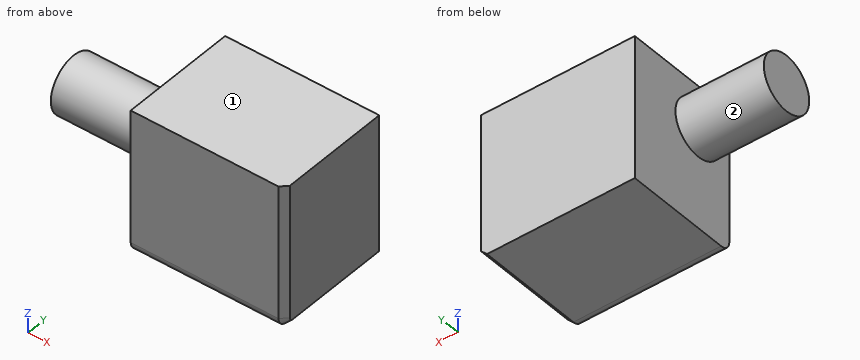
```python
from build123d import *

# Parameters (mm, degrees)
F0_W     = 125.304118
F0_H     = 116.59091
F1_DEPTH = 95.108278
F2_R     = 8.21097
F3_SIZE  = 5.08
F4_R     = 22.853538
F5_DEPTH = 71.891591


with BuildPart() as f1:
    # F0 (on Front) → F1 (new body)
    with BuildSketch(Plane.XZ):
        with Locations((1.244716, -1.867104)):
            Rectangle(F0_W, F0_H)
    extrude(amount=F1_DEPTH)

    # F2
    f2_edges = [f1.edges().sort_by_distance(p)[0] for p in [
        (1.244716, -95.108278, -60.162559),
    ]]
    fillet(f2_edges, radius=F2_R)

    # F3
    f3_edges = [f1.edges().sort_by_distance(p)[0] for p in [
        (63.896775, -95.108278, 2.238381),
    ]]
    chamfer(f3_edges, length=F3_SIZE)

    # F4 (on face) → F5 (join)
    with BuildSketch(Plane(origin=(-61.407343, 0, 0), x_dir=(0, -1, 0), z_dir=(-1, 0, 0))):
        with Locations((63.728884, 21.200262)):
            Circle(F4_R)
    extrude(amount=F5_DEPTH)


solid = f1.part
```
The listing builds one solid part. Answer for the finished solid, in the listing's coordinates (mm). Face numbers are marked on the shaded views. A direction names the side the tool comes from. Coordinates: 2 decimals unless noted, no trailing zeros. Write each loop counter-clockwise with the first axis right and the second up, starting at its lowest first coordinate (ties: lowest second). Pieces come first, ordered by that corner, then holes. Notation, with made-up numbers: M 46,14 L 62,14 A24 ccw 62,43 Z; hole C -37.75,42.25 d1. An arc over 180 degrees is marked long. Use a Markdown table: item, result. Add a question column.
1. Straight lines are drawn through the part: line 1 along X through (y, z) = (-38, 20.5); line 2 along Z through (x, y) = (-73.5, -64); line 3 along Y through (x, z) = (-117, 12). For each, find the intervals that lie inside material, in ascending order. Write a range as [from, to].
2. Section A-A (z = 34) is taken. Give the vertices of the cut face in (x, y).
3. Section C-C (x = -95) is taken. Give the vertices of the cut face in (y, z), plus the area to 3 significant figures.
4. Section D-D (z = 15) is taken. Give the vertices of the cut face in (x, y).
5. Which of the six approach directions +Z, -Z, +X, -X, +Y, -Y give full straight-line access (tool end or side, diameter ignored) to the marked faces 1 and 2?
6. Given P1, Ø3, axis at x = -88, z = 19.5, coming from the +Y side; P2, Ø12, axis at y = -63, z = -24, coming from the -X side, each flat-ended and moving along its own axis, determine where each tip first touches the part or whether it passes through.
7. Section B-B (y = -6.5) is taken. Give the vertices of the cut face in (x, z).
Data:
| question | item | result |
|---|---|---|
| 1 | line 1 | x = [-61.41, 63.9] |
| 1 | line 2 | z = [-1.65, 44.05] |
| 1 | line 3 | y = [-84.65, -42.81] |
| 2 | outline | M -133.3,-82.66 L -61.41,-82.66 L -61.41,-95.11 L 58.82,-95.11 L 63.9,-90.03 L 63.9,0 L -61.41,0 L -61.41,-44.8 L -133.3,-44.8 Z |
| 3 | outline | C -63.73,21.2 d45.71 |
| 3 | area | 1,640 mm2 |
| 4 | outline | M -133.3,-85.73 L -61.41,-85.73 L -61.41,-95.11 L 58.82,-95.11 L 63.9,-90.03 L 63.9,0 L -61.41,0 L -61.41,-41.73 L -133.3,-41.73 Z |
| 5 | face 1 | +Z, +X, -X, +Y, -Y |
| 5 | face 2 | -X |
| 6 | P1 | stops at y = -40.88 |
| 6 | P2 | stops at x = -61.41 |
| 7 | outline | M -61.41,-60.16 L 58.82,-60.16 L 63.9,-55.08 L 63.9,56.43 L -61.41,56.43 Z |
